```python
from build123d import *

# Parameters (mm, degrees)
F1_DEPTH = 50


# Not quite as in the source:
# - ends of sketch curves that miss each other by under 0.0002 mm in the source are joined


with BuildPart() as f1:
    # F0 (on Front) → F1 (new body)
    with BuildSketch(Plane.XZ):
        with BuildLine():
            Line((-719.030741, 535.802017), (-716.260339, 551.935195))
            Line((-716.260339, 551.935195), (-735.912365, 548.229318))
            ThreePointArc((-735.912365, 548.229318), (-818.0414227516, 477.1771162339), (-814.0615494377, 368.65173577))
            ThreePointArc((-814.0615494377, 368.65173577), (-813.3377138775, 356.2962207865), (-822.1469540915, 347.602546248))
            Line((-822.1469540915, 347.602546248), (-837.503896, 341.935195))
            Line((-837.503896, 341.935195), (-824.468499, 326.76898))
            ThreePointArc((-824.468499, 326.76898), (-721.8709589722, 291.1692315288), (-629.8751597113, 348.8785918176))
            ThreePointArc((-629.8751597113, 348.8785918176), (-619.5368877345, 355.6832101227), (-607.6033241523, 352.4010218168))
            Line((-607.6033241523, 352.4010218168), (-595.016783, 341.935195))
            Line((-595.016783, 341.935195), (-588.400154, 360.807287))
            ThreePointArc((-588.400154, 360.807287), (-608.868637199, 467.4592376194), (-704.8443090013, 518.2752569674))
            ThreePointArc((-704.8443090013, 518.2752569674), (-715.9064175677, 523.8261534239), (-719.030741, 535.802017))
        make_face()
        Polygon((-767.376564, 415.399297), (-744.818452, 454.471094), (-738.818452, 457.935195), (-693.702227, 457.935195), (-687.702227, 454.471094), (-665.144115, 415.399297), (-665.144115, 408.471094), (-687.702227, 369.399297), (-693.702227, 365.935195), (-738.818452, 365.935195), (-744.818452, 369.399297), (-767.376564, 408.471094), align=None, mode=Mode.SUBTRACT)
    extrude(amount=F1_DEPTH)


solid = f1.part
```
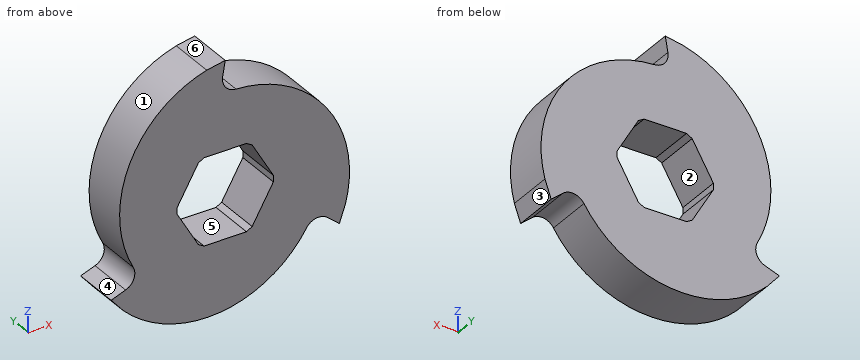
Model file for the job. Use its own axes, mm. Face numbers are marked on the shaded views. A direction names the side the tool comes from. Give positions to 0.01 mm unless a question says otherwise; leave off trailing zeros. Loops run counter-clockwise (first coordinate to the right, second up) from the corner with the lowest first, then second, coordinate; pieces in that order, holes last. Notation, with made-up numbers: (8.5, -24.5) - (35.5, -24.5) arc R16 ccw to (35.5, -0.5) - close; hole circle Ø1 at (-21, 11). An arc over 180 degrees is marked (long way). One line per item, written item: value. Start each with the question number.
1. Slice it at D-D (x = -633.5). List the corners of the cut face in (y, z), plus the area to 3 significant figures.
2. Slice it at A-A (x = -678.5). List the corners of the cut face in (y, z), plus the area to 3 significant figures.
3. Slice it at C-C (z = 441). List the corners of the cut face in (x, y), plus the area to 3 significant figures.
4. Pull direction X, two halves, no side cores. Call the marked faces 1, 2 and 3: pulls with the +X half, pulls with the -X half, needs draft (parallel to the pull), parting line crosses it, or undercut.
5. Which spindle directions (+Z, -Z, +X, -X, +Y, -Y) get a long thin tool onto all of the face, cutting with end or side? Do the marked faces 4, 5 and 6. Say none if no direction does.
6. Pin check, flat tips, straight feed: pin 1 (22.5 mm diameter, centred on x = -727, y = -29.5, fed in from -Z); pin 2 (10 mm diameter, centred on y = -30, z = 340.5, fed in from +X); pin 3 (13.5 mm diameter, centred on x = -707.5, y = -29.5, fed in from +Z). Stop position of each tip, or through.
7. Slice it at B-B (y = -7.5). List the corners of the cut face in (x, z), plus the area to 3 significant figures.
8. Probe L1, parallel to Z at x = -684, y = -10; L2, parallel to X at y = -39, z = 455.5; L3, parallel to Z at x = -760, y = -33.5. List the from-to ranges inside material, lowest first. Write a range as from..to.
Solution:
1. outline: (-50, 343.46) - (0, 343.46) - (0, 492.51) - (-50, 492.51) - close
1. area: 7,450 mm^2
2. outline: (-50, 304.33) - (0, 304.33) - (0, 385.34) - (-50, 385.34) - close; (-50, 438.53) - (0, 438.53) - (0, 514.4) - (-50, 514.4) - close
2. area: 7,840 mm^2
3. outline: (-827.7, -50) - (-752.6, -50) - (-752.6, 0) - (-827.7, 0) - close; (-679.92, -50) - (-593.88, -50) - (-593.88, 0) - (-679.92, 0) - close
3. area: 8,060 mm^2
4. face 1: pulls with the -X half
4. face 2: undercut
4. face 3: pulls with the +X half
5. face 4: -X, +Y, -Y
5. face 5: +Y, -Y
5. face 6: +Z, -X, +Y, -Y
6. pin 1: stops at z = 290.37
6. pin 2: stops at x = -593.77
6. pin 3: stops at z = 522.09
7. outline: (-837.5, 341.94) - (-824.47, 326.77) arc R125.58 ccw to (-629.88, 348.88) arc R15 cw to (-607.6, 352.4) - (-595.02, 341.94) - (-588.4, 360.81) arc R125.58 ccw to (-704.84, 518.28) arc R15 cw to (-719.03, 535.8) - (-716.26, 551.94) - (-735.91, 548.23) arc R125.58 ccw to (-814.06, 368.65) arc R15 cw to (-822.15, 347.6) - close; hole (-767.38, 408.47) - (-744.82, 369.4) - (-738.82, 365.94) - (-693.7, 365.94) - (-687.7, 369.4) - (-665.14, 408.47) - (-665.14, 415.4) - (-687.7, 454.47) - (-693.7, 457.94) - (-738.82, 457.94) - (-744.82, 454.47) - (-767.38, 415.4) - close
7. area: 39,100 mm^2
8. L1: z = 301.66..375.81, 448.06..515.69
8. L2: x = -825.21..-743.04, -689.48..-601.04
8. L3: z = 292.67..395.69, 428.18..538.91
